```python
from build123d import *

# Parameters (mm, degrees)
SKETCH4_W           = 30
SKETCH4_H           = 20
SKETCH4_R           = 1
BOSS_EXTRUDE2_DEPTH = 1.5


with BuildPart() as part:
    # Sketch4 → Boss-Extrude2 (new body)
    with BuildSketch(Plane.XY):
        with Locations((2.769964864, 12.5155541)):
            Rectangle(SKETCH4_W, SKETCH4_H)
        with Locations((-4.730035136, 5.0155541)):
            Circle(SKETCH4_R, mode=Mode.SUBTRACT)
        with Locations((15.269964864, 5.0155541)):
            Circle(SKETCH4_R, mode=Mode.SUBTRACT)
        with BuildLine():
            Line((-6.230035136, 18.5155541), (11.769964864, 18.5155541))
            ThreePointArc((11.769964864, 18.5155541), (12.769964864, 17.5155541), (11.769964864, 16.5155541))
            Line((11.769964864, 16.5155541), (-6.230035136, 16.5155541))
            ThreePointArc((-6.230035136, 16.5155541), (-7.230035136, 17.5155541), (-6.230035136, 18.5155541))
        make_face(mode=Mode.SUBTRACT)
    extrude(amount=BOSS_EXTRUDE2_DEPTH)


solid = part.part
```
Geometry check sheet. Reference: the model listing, model coordinates, mm. A direction names the side the tool comes from. Give positions to 0.01 mm unless a question says otherwise; leave off trailing zeros. Order: outer loops, then holes, each group sorted by start corner. A loop starts at its lowest first (then second) coordinate and runs counter-clockwise, first axis right, second up. Notation, with made-up numbers: (-35, -39) - (-16, -39) arc R6 cw to (-16, -34) - close; hole circle Ø2 at (-8.75, -9.5). An arc over 180 degrees is marked (long way). Write item = value, one per line. Start each with the question number.
1) Draft check along X on faces 1 (the flat face through (3, 13, 1.5)), 2 (the flat face through (3, 18.516, 1)), 3 (the flat face through (17.77, 12, 1)). Enter one of: released by +X, released by -X, zero draft, split by the parting line, or undercut.
2) Access from +Z, -Z, +X, -X, +Y, -Y to the whole of each face (thin tool, end or side, straight path). Record for faces 4 (the flat face through (-12.23, 12, 1)), 5 (the cylindrical face through (12.77, 17.54, 0.74)).
3) Section check C-C (y = 4.5). Enter the section's corners in (x, z).
4) Section check D-D (z = 0.55). Enter the section's corners in (x, y).
5) Gauge pin test, flat end, axial feed: pin 1 Ø1.6 at (x, y) = (15.27, 5.02) entering from +Z. Record the tip position at first contact, or that the pin passes through.
6) Section check B-B (x = -4.5). Enter the section's corners in (y, z).
7) Section check A-A (x = 7.25). Enter the section's corners in (y, z).
8) Scan lines: L1, parallel to Y at x = 1, z = 0.3; L2, parallel to X at y = 17.5, z = 0.2; L3, parallel to X at y = 4.75, z = 1.1. Record each from-to range of solid material in increasing order.
Geometry check:
q1.face_1 = zero draft
q1.face_2 = undercut
q1.face_3 = released by +X
q2.face_4 = +Z, -Z, -X, +Y, -Y
q2.face_5 = +Z, -Z
q3.outline = (-12.23, 0) - (-5.59, 0) - (-5.59, 1.5) - (-12.23, 1.5) - close; (-3.87, 0) - (14.41, 0) - (14.41, 1.5) - (-3.87, 1.5) - close; (16.13, 0) - (17.77, 0) - (17.77, 1.5) - (16.13, 1.5) - close
q4.outline = (-12.23, 2.52) - (17.77, 2.52) - (17.77, 22.52) - (-12.23, 22.52) - close; hole (-6.23, 16.52) - (11.77, 16.52) arc R1 ccw to (11.77, 18.52) - (-6.23, 18.52) arc R1 ccw to start; hole circle Ø2 at (-4.73, 5.02); hole circle Ø2 at (15.27, 5.02)
q5.pin_1 = through
q6.outline = (2.52, 0) - (4.04, 0) - (4.04, 1.5) - (2.52, 1.5) - close; (5.99, 0) - (16.52, 0) - (16.52, 1.5) - (5.99, 1.5) - close; (18.52, 0) - (22.52, 0) - (22.52, 1.5) - (18.52, 1.5) - close
q7.outline = (2.52, 0) - (16.52, 0) - (16.52, 1.5) - (2.52, 1.5) - close; (18.52, 0) - (22.52, 0) - (22.52, 1.5) - (18.52, 1.5) - close
q8.L1 = 2.52 to 16.52, 18.52 to 22.52
q8.L2 = -12.23 to -7.23, 12.77 to 17.77
q8.L3 = -12.23 to -5.69, -3.77 to 14.31, 16.23 to 17.77
